```python
from build123d import *

# Parameters (mm, degrees)
SKETCH_1_R          = 8
SKETCH_1_R_2        = 4.5
EXTRUDE_1_DEPTH     = 4
CUT_EXTRUDE_2_DEPTH = 221.943431674
SKETCH_3_R          = 1.7
CUT_EXTRUDE_3_DEPTH = 221.943431674


with BuildPart() as part:
    # 草图1 → 凸台-拉伸1 (new body)
    with BuildSketch(Plane.XY):
        with BuildLine():
            Line((-20, 0), (-20, -200))
            ThreePointArc((-20, -200), (0, -220), (20, -200))
            Line((20, -200), (20, 0))
            ThreePointArc((20, 0), (0, 20), (-20, 0))
        make_face()
        Circle(SKETCH_1_R, mode=Mode.SUBTRACT)
        with Locations((0, -200)):
            Circle(SKETCH_1_R_2, mode=Mode.SUBTRACT)
    extrude(amount=EXTRUDE_1_DEPTH)

    # 草图2 → 切除-拉伸2 (cut, through all)
    with BuildSketch(Plane.XY.offset(4)):
        with BuildLine():
            Line((-5, -31.845004689), (-5, -159.845004689))
            ThreePointArc((-5, -159.845004689), (0, -164.845004689), (5, -159.845004689))
            Line((5, -159.845004689), (5, -31.845004689))
            ThreePointArc((5, -31.845004689), (0, -26.845004689), (-5, -31.845004689))
        make_face()
    extrude(amount=-CUT_EXTRUDE_2_DEPTH, mode=Mode.SUBTRACT)

    # 草图3 → 切除-拉伸3 (cut, through all)
    with BuildSketch(Plane(origin=(0, 0, 0), x_dir=(-1, 0, 0), z_dir=(0, 0, -1))):
        with Locations((0, -214)):
            Circle(SKETCH_3_R)
        with Locations((-12.124355653, -193)):
            Circle(SKETCH_3_R)
        with Locations((12.124355653, -193)):
            Circle(SKETCH_3_R)
    extrude(amount=-CUT_EXTRUDE_3_DEPTH, mode=Mode.SUBTRACT)


solid = part.part
```
Verification items for the finished model (mm, model axes). A direction names the side the tool comes from. Give positions to 0.01 mm unless a question says otherwise; leave off trailing zeros. Order: outer loops, then holes, each group sorted by start corner. A loop starts at its lowest first (then second) coordinate and runs counter-clockwise, first axis right, second up. Notation, with made-up numbers: (26.25, -13) -> (60.25, -13) arc R13 cw to (60.25, -8) -> close; hole circle Ø11 at (82.25, 20). An arc over 180 degrees is marked (long way). One line per item, written item: value.
(1) Sectioned sample at B-B on z = 0.6. Record the cut outline in (x, y) (3 decimals), then the cut area to 3 significant figures.
Final values:
outline: (-20, -200) arc R20 ccw to (20, -200) -> (20, 0) arc R20 ccw to (-20, 0) -> close; hole circle Ø3.4 at (-12.124, -193); hole circle Ø16 at (0, 0); hole (-5, -159.845) arc R5 ccw to (5, -159.845) -> (5, -31.845) arc R5 ccw to (-5, -31.845) -> close; hole circle Ø9 at (0, -200); hole circle Ø3.4 at (0, -214); hole circle Ø3.4 at (12.124, -193)
area: 7,610 mm^2
(2) Draft check along X on faces 1 (the face through (-1.73, -7.81, 1.97)), 2 (the face through (20, -101, 2)), 3 (the face through (9, -98, 4)), 4 (the face through (-5, -95, 2)). Enter one of: pulls with the +X half, pulls with the -X half, needs draft (parallel to the pull), parting line crosses it, or undercut.
Final values:
face 1: undercut
face 2: pulls with the +X half
face 3: needs draft
face 4: undercut
(3) Tool access check on faces 5 (the face through (-20, -99, 2)), 6 (the face through (0.11, -26.846, 2.028)). Record the directions out of +Z, -Z, +X, -X, +Y, -Y that give a thin tool (end or side, any length) a straight path to the whole face; none if there is none.
Final values:
face 5: +Z, -Z, -X, +Y, -Y
face 6: +Z, -Z
(4) Sectioned sample at A-A on y = -82. Record the cut outline in (x, z), then the cut area to 3 significant figures.
Final values:
outline: (-20, 0) -> (-5, 0) -> (-5, 4) -> (-20, 4) -> close; (5, 0) -> (20, 0) -> (20, 4) -> (5, 4) -> close
area: 120 mm^2
(5) Sectioned sample at C-C on x = 16.5. Record the cut outline in (y, z), then the cut area to 3 significant figures.
Final values:
outline: (-211.3, 0) -> (11.3, 0) -> (11.3, 4) -> (-211.3, 4) -> close
area: 890 mm^2
(6) Scan lines: line 1 along X through (y, z) = (-193, 1.85); line 2 along Y through (x, z) = (0, 2.8) (3 decimals); line 3 along X through (y, z) = (-77, 0.65). Record each from-to range of solid material in increasing order. Write a range as [from, to].
Final values:
line 1: [-20, -13.82], [-10.42, 10.42], [13.82, 20]
line 2: [-220, -215.7], [-212.3, -204.5], [-195.5, -164.845], [-26.845, -8], [8, 20]
line 3: [-20, -5], [5, 20]
